Verification items for this drawing (mm, ordinates from the low corner). Round coordinates to 2 decimals unless told otherwise and drop trailing zeros. Loops run counter-clockwise (first coordinate to the right, second up) from the corner with the lowest first, then second, coordinate; pieces in that order, holes last. Notation, with made-up numbers: M 34.25,31.25 L 72.25,31.25 A19 ccw 72.25,58.25 Z; hole C 67,48 d8. An arc over 180 degrees is marked long. Use one line per item in the form item = value. Start each with the question number.
1. Material ranges on line 1 (Z direction, x = 240.5, y = 273); line 2 (Z direction, x = 306.5, y = 286); line 3 (Z direction, x = 147.5, y = 127.5), recorded low to high.
2. Cross-section at B-B (y = 163.5). Record the boundary of the cut face in (x, z).
3. Cross-section at A-A (x = 344). Record the boundary of the cut face in (y, z).
4. Go/stop test with a flat-tipped pin: pin 1 (12 mm diameter, centred on x = 201.5, y = 215, fed in from +Z). Record where the tip stops, or that it passes through.
5. Cross-section at C-C (z = 722.5). Record the boundary of the cut face in (x, y).
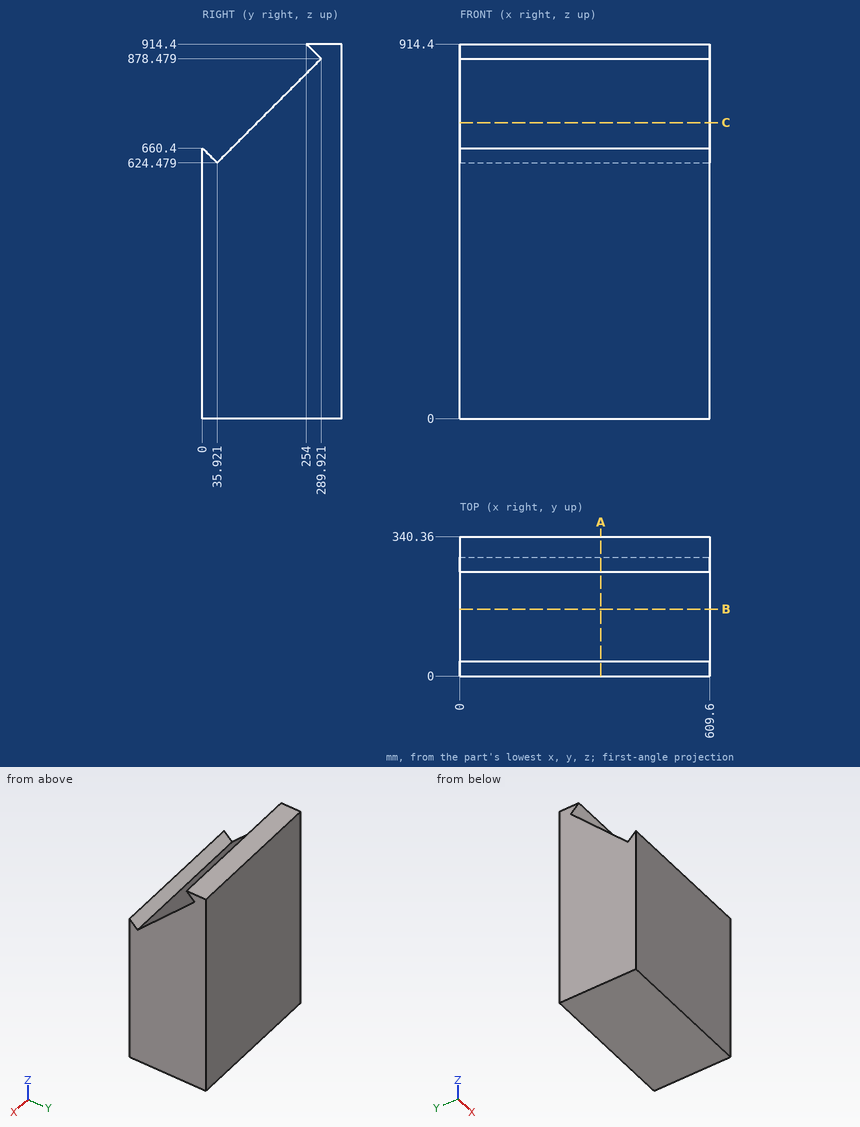
Reported:
q1.line_1 = 0 to 861.56, 895.4 to 914.4
q1.line_2 = 0 to 874.56, 882.4 to 914.4
q1.line_3 = 0 to 716.06
q2.outline = M 0,0 L 609.6,0 L 609.6,752.06 L 0,752.06 Z
q3.outline = M 0,0 L 340.36,0 L 340.36,914.4 L 254,914.4 L 289.92,878.48 L 35.92,624.48 L 0,660.4 Z
q4.pin_1 = 809.56
q5.outline = M 0,133.94 L 609.6,133.94 L 609.6,340.36 L 0,340.36 Z
